from build123d import *

# Parameters (mm, degrees)
BOSS_EXTRUDE1_DEPTH     = 3.175
CUT_EXTRUDE1_DEPTH      = 65.189801711
CUT_EXTRUDE1_DEPTH_BACK = 65.189801711
SKETCH3_R               = 1.35
SKETCH3_R_2             = 1.397
SKETCH5_W               = 6
SKETCH5_H               = 4.2
CUT_EXTRUDE2_DEPTH      = 65.189801711


with BuildPart() as part:
    # Sketch2 → Boss-Extrude1 (new body)
    with BuildSketch(Plane(origin=(0, 0, 0), x_dir=(1, 0, 0), z_dir=(0, 1, 0))):
        with BuildLine():
            Line((48, 42.5), (-48, 42.5))
            Line((-48, 42.5), (-48, -10.75))
            add(Edge.make_bspline(
                [(-48, -10.75), (-48, -53.083333333), (48, -53.083333333), (48, -10.75)],
                knots=[0, 0, 0, 0, 1, 1, 1, 1], degree=3))
            Line((48, -10.75), (48, 42.5))
        make_face()
    extrude(amount=BOSS_EXTRUDE1_DEPTH)

    # Sketch3 → Cut-Extrude1 (cut, two sides: drawn at the far end of the back side and taken through both)
    with BuildSketch(Plane(origin=(0, 3.175, 0), x_dir=(1, 0, 0), z_dir=(0, 1, 0)).offset(-CUT_EXTRUDE1_DEPTH_BACK)):
        with Locations(Location((-30, 19.5, 0), (0, 0, 270))):
            Circle(SKETCH3_R)
        with Locations(Location((-30, -25.5, 0), (0, 0, 270))):
            Circle(SKETCH3_R)
        with Locations(Location((30, -25.5, 0), (0, 0, 90))):
            Circle(SKETCH3_R)
        with Locations(Location((30, 19.5, 0), (0, 0, 90))):
            Circle(SKETCH3_R)
        with Locations(Location((-23, 12.5, 0), (0, 0, 270))):
            Circle(SKETCH3_R_2)
        with Locations(Location((-23, -10.5, 0), (0, 0, 270))):
            Circle(SKETCH3_R_2)
        with Locations(Location((35, -10.5, 0), (0, 0, 90))):
            Circle(SKETCH3_R_2)
        with Locations(Location((35, 12.5, 0), (0, 0, 90))):
            Circle(SKETCH3_R_2)
    extrude(amount=CUT_EXTRUDE1_DEPTH + CUT_EXTRUDE1_DEPTH_BACK, mode=Mode.SUBTRACT)

    # Sketch5 → Cut-Extrude2 (cut, through all)
    with BuildSketch(Plane(origin=(0, 3.175, 0), x_dir=(1, 0, 0), z_dir=(0, 1, 0))):
        with Locations((24.051144599, 40.4)):
            Rectangle(SKETCH5_W, SKETCH5_H)
        with Locations((-23.948855401, 40.4)):
            Rectangle(SKETCH5_W, SKETCH5_H)
    extrude(amount=-CUT_EXTRUDE2_DEPTH, mode=Mode.SUBTRACT)


solid = part.part
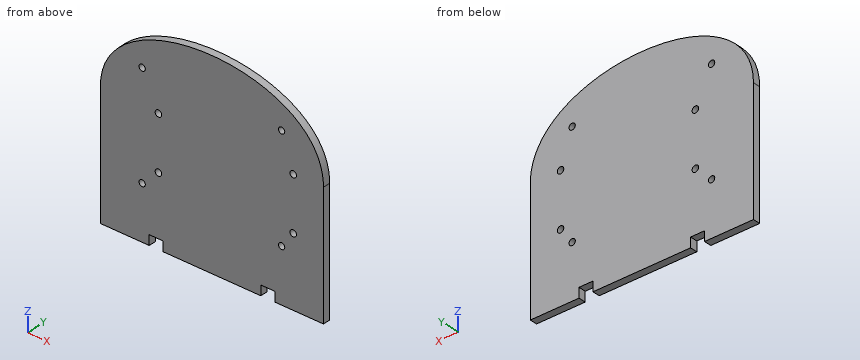
The listing builds one solid part. Answer for the finished solid, in the listing's coordinates (mm). Round coordinates to 2 decimals unless told otherwise and drop trailing zeros. Order: outer loops, then holes, each group sorted by start corner. A loop starts at its lowest first (then second) coordinate and runs counter-clockwise, first axis right, second up. Notation, with made-up numbers: (4.5, -34) -> (55.5, -34) arc R20 ccw to (55.5, -14) -> close; hole circle Ø5 at (54, -2). An arc over 180 degrees is marked (long way). One line per item, written item: value.
Item 1: Straight lines are drawn through the part: L1, parallel to X at y = 2.3, z = -12.5; L2, parallel to X at y = 2, z = -19.5; L3, parallel to Z at x = -30, y = 1.25. For each, find the intervals that lie inside material, in ascending order.
Taken from the geometry:
L1: x = -48 to -24.4, -21.6 to 33.6, 36.4 to 48
L2: x = -48 to -31.35, -28.65 to 28.65, 31.35 to 48
L3: z = -42.5 to -20.85, -18.15 to 24.15, 26.85 to 36.18
Item 2: Find section A-A, the plane z = -12.5. Give the vertices of the cut face in (x, y) (3 decimals), then the cut area to 3 significant figures.
Taken from the geometry:
outline: (-48, 0) -> (-24.397, 0) -> (-24.397, 3.175) -> (-48, 3.175) -> close; (-21.603, 0) -> (33.603, 0) -> (33.603, 3.175) -> (-21.603, 3.175) -> close; (36.397, 0) -> (48, 0) -> (48, 3.175) -> (36.397, 3.175) -> close
area: 287 mm2
Item 3: Find section B-B, the plane y = 1.8. State how many separate pieces and enclosed holes the cut face has, then the cut area to 3 significant figures.
Taken from the geometry:
separate pieces: 1
enclosed holes: 8
area: 7,450 mm2
Item 4: Given P1, Ø4.5, axis at x = -23, z = -12.5, coming from the +Y side (3 decimals); P2, Ø1, axis at x = 37.5, y = 1.5, coming from the +Z side; P3, Ø1, axis at x = 23, y = 2, coming from the -Z side, each flat-ended and moving along its own axis, determine where each tip first touches the part or whether it passes through.
Taken from the geometry:
P1: stops at y = 3.175
P2: stops at z = 31.88
P3: stops at z = -38.3
